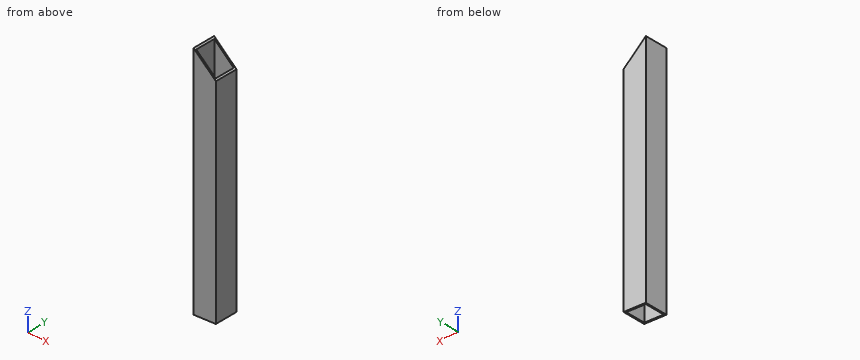
```python
from build123d import *

# Parameters (mm, degrees)
SKETCH1_W           = 25.4
SKETCH1_H           = 25.4
SKETCH1_W_2         = 22.098
SKETCH1_H_2         = 22.098
BOSS_EXTRUDE1_DEPTH = 252.579
SKETCH5_W           = 25.4
SKETCH5_H           = 25.4
SKETCH5_W_2         = 22.098
SKETCH5_H_2         = 22.098
BOSS_EXTRUDE2_DEPTH = 12.7
CUT_EXTRUDE1_DEPTH  = 36.4
SKETCH7_W           = 25.4
SKETCH7_H           = 25.4
SKETCH7_W_2         = 22.098
SKETCH7_H_2         = 22.098
BOSS_EXTRUDE3_DEPTH = 25.4
CUT_EXTRUDE2_DEPTH  = 165.021579309


with BuildPart() as part:
    # Sketch1 → Boss-Extrude1 (new body)
    with BuildSketch(Plane.XY):
        Rectangle(SKETCH1_W, SKETCH1_H)
        Rectangle(SKETCH1_W_2, SKETCH1_H_2, mode=Mode.SUBTRACT)
    extrude(amount=BOSS_EXTRUDE1_DEPTH)

    # Sketch5 → Boss-Extrude2 (add)
    with BuildSketch(Plane.XY.offset(252.579)):
        Rectangle(SKETCH5_W, SKETCH5_H)
        Rectangle(SKETCH5_W_2, SKETCH5_H_2, mode=Mode.SUBTRACT)
    extrude(amount=BOSS_EXTRUDE2_DEPTH)

    # Sketch6 → Cut-Extrude1 (cut, through all)
    with BuildSketch(Plane(origin=(0, -22.7, 252.579), x_dir=(-0.142456183, 0, 0.989801109), z_dir=(0, -1, 0))):
        Polygon((-25.049344305, -21.702249197), (26.869925532, 23.279564235), (45.864950848, -41.551460554), align=None)
    extrude(amount=-CUT_EXTRUDE1_DEPTH, mode=Mode.SUBTRACT)

    # Sketch7 → Boss-Extrude3 (add)
    with BuildSketch(Plane(origin=(0, 0, 0), x_dir=(-1, 0, 0), z_dir=(0, 0, -1))):
        Rectangle(SKETCH7_W, SKETCH7_H)
        Rectangle(SKETCH7_W_2, SKETCH7_H_2, mode=Mode.SUBTRACT)
    extrude(amount=BOSS_EXTRUDE3_DEPTH)

    # Sketch8 → Cut-Extrude2 (cut, through all)
    with BuildSketch(Plane(origin=(602.971957407, 151.321579309, -52.668394102), x_dir=(0.142456183, 0, -0.989801109), z_dir=(0, -1, 0))):
        Polygon((-136.208901871, -563.906106683), (-139.847734949, -614.732641149), (-41.725602435, -599.280432209), align=None)
    extrude(amount=CUT_EXTRUDE2_DEPTH, mode=Mode.SUBTRACT)


solid = part.part
```
Geometry check sheet. Reference: the model listing, model coordinates, mm. Coordinates: 2 decimals unless noted, no trailing zeros. Order: outer loops, then holes, each group sorted by start corner. A loop starts at its lowest first (then second) coordinate and runs counter-clockwise, first axis right, second up. Notation, with made-up numbers: (15.5, 68.25) - (59.5, 68.25) arc R14 cw to (59.5, 87.25) - close; hole circle Ø5 at (3.5, 32). An arc over 180 degrees is marked (long way). Answer as a JSON object with one key per item and string values. Group by question number.
Item 1: Sectioned sample at A-A, the plane y = 4.25. Record the cut outline in (x, z), and give its area (3 significant figures).
Item 2: Sectioned sample at C-C, the plane x = -0.25. Record the cut outline in (y, z), and give its area (3 significant figures).
Item 3: Sectioned sample at B-B, the plane z = 21. Record the cut outline in (x, y), and give its area (3 significant figures).
Item 4: Scan line: probe 1 along Y at (x, z) = (-7.75, 40). Record every from-to range of solid material in increasing order.
Resolved:
{
 "1": {"outline": "(-12.7, -0.91) - (-11.05, -0.79) - (-11.05, 262.15) - (-12.7, 263.58) - close; (11.05, 0.79) - (12.7, 0.91) - (12.7, 241.58) - (11.05, 243.01) - close", "area": "834 mm^2"},
 "2": {"outline": "(-12.7, -0.02) - (-11.05, -0.02) - (-11.05, 252.8) - (-12.7, 252.8) - close; (11.05, -0.02) - (12.7, -0.02) - (12.7, 252.8) - (11.05, 252.8) - close", "area": "835 mm^2"},
 "3": {"outline": "(-12.7, -12.7) - (12.7, -12.7) - (12.7, 12.7) - (-12.7, 12.7) - close; hole (-11.05, -11.05) - (11.05, -11.05) - (11.05, 11.05) - (-11.05, 11.05) - close", "area": "157 mm^2"},
 "4": {"probe 1": "-12.7 to -11.05, 11.05 to 12.7"}
}
